Part model, mm, in its own coordinate system. Face numbers are marked on the shaded views. A direction names the side the tool comes from. Round coordinates to 2 decimals unless told otherwise and drop trailing zeros. Loops run counter-clockwise (first coordinate to the right, second up) from the corner with the lowest first, then second, coordinate; pieces in that order, holes last.
from build123d import *

# Parameters (mm, degrees)
F1_DEPTH = 32
F3_DEPTH = 32


with BuildPart() as f1:
    # F0 (on Front) → F1 (new body)
    with BuildSketch(Plane.XZ):
        Polygon((-38, -55.5), (-38, -61.5), (38, -61.5), (38, -55.5), (20, -55.5), (5, -55.5), (-5, -55.5), (-20, -55.5), align=None)
        Polygon((-5, 34.5), (-5, -55.5), (5, -55.5), (5, 34.5), (5, 61.5), (-5, 61.5), align=None)
    extrude(amount=F1_DEPTH)

    # F2 (on Front) → F3 (join)
    with BuildSketch(Plane.XZ):
        with BuildLine():
            Line((5, -55.5), (20, -55.5))
            add(Edge.make_bspline(
                [(5, 34.5), (9, -21.117978), (11, -41.342697), (20, -55.5)],
                knots=[0, 0, 0, 0, 1, 1, 1, 1], degree=3))
            Line((5, 34.5), (5, -55.5))
        make_face()
        with BuildLine():
            add(Edge.make_bspline(
                [(-5, 34.5), (-9, -21.117978), (-11, -41.342697), (-20, -55.5)],
                knots=[0, 0, 0, 0, 1, 1, 1, 1], degree=3))
            Line((-20, -55.5), (-5, -55.5))
            Line((-5, -55.5), (-5, 34.5))
        make_face()
    extrude(amount=F3_DEPTH)


solid = f1.part
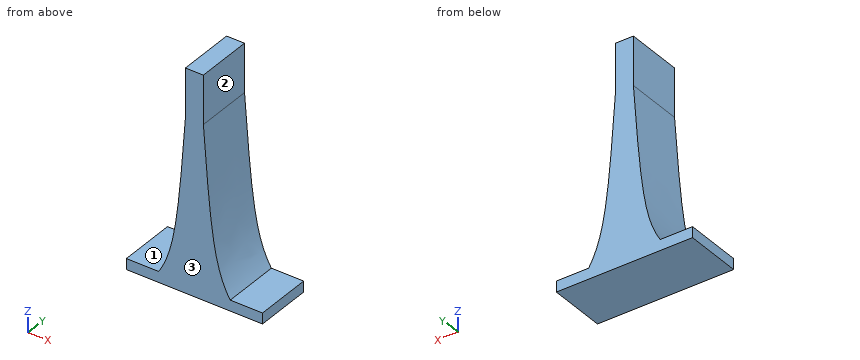
1) Slice it at A-A, the plane x = 27. Give the cut face in (y, z), then the cut area to 3 significant figures.
Values:
outline: (-32, -61.5) - (0, -61.5) - (0, -55.5) - (-32, -55.5) - close
area: 192 mm2
2) Drop flat-ended pins along their axis: pin 1 Ø14.5 at (x, y) = (25.5, -20.5) entering from +Z; pin 2 Ø1 at (x, y) = (16.5, -24.5) entering from +Z; pin 3 Ø6 at (x, z) = (-9, 48.5) entering from +Y; pin 4 Ø2 at (y, z) = (-25.5, 21) entering from +X. Give the stop position or say it passes through.
Values:
pin 1: stops at z = -52.5
pin 2: stops at z = -47.68
pin 3: passes through
pin 4: stops at x = 6.06
3) Wall check: line 1 along Z through (x, y) = (33, -27); line 2 along X through (y, z) = (-13.5, 47); line 3 along X through (y, z) = (-19.5, 22). Give the ranges that are in metal, low to high.
Values:
line 1: z = -61.5 to -55.5
line 2: x = -5 to 5
line 3: x = -5.91 to 5.91
4) Tool access for the marked faces 1, 2 and 3: list every direction of +Z, -Z, +X, -X, +Y, -Y with a clear straight run to the whole face (end or side of a thin tool).
Values:
face 1: +Z, -X, +Y, -Y
face 2: +Z, +X, +Y, -Y
face 3: +Z, -Z, +X, -X, -Y
